The drawing under review shows one solid part. Ordinate dimensions are in mm from its lowest x, y, z. A direction names the side the tool comes from. Coordinates: 2 decimals unless noted, no trailing zeros. Write each loop counter-clockwise with the first axis right and the second up, starting at its lowest first coordinate (ties: lowest second). Pieces come first, ordered by that corner, then holes. Notation, with made-up numbers: M -1.5,-26.5 L 21.5,-26.5 A21 cw 21.5,-12.5 Z; hole C 10.5,19 d9. An arc over 180 degrees is marked long. Write each question's results on one line, items separated by ' | '. Start each with the question number.
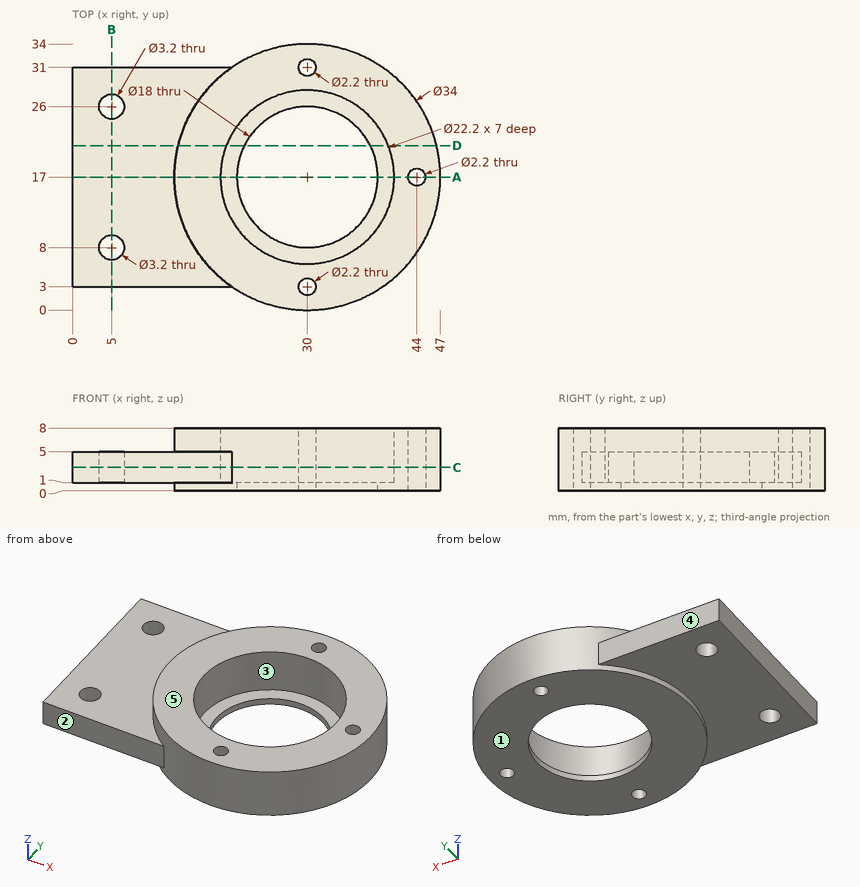
Item 1: For the marked faces 4 and 5, list the 3-axis set-ups (+Z, -Z, +X, -X, +Y, -Y) from which the entire face can be reached by the end or side of a thin tool; tool diameter is ignored.
Item 2: We need section A-A on y = 17. State the section outline as (x, z) points, then the cut area to 3 significant figures.
Item 3: We need section D-D on y = 21. State the section outline as (x, z) points.
Item 4: Draft analysis for pull direction Y (two halves, no side actions). For the marked faces 1, 2 and 3, state which applies: released by +Y, released by -Y, zero draft, split by the parting line, or undercut.
Item 5: Insertion check: pin 1 Ø1.5 at (y, z) = (20.5, 3.5) entering from +X; pin 2 Ø11 at (x, y) = (25.5, 14) entering from +Z; pin 3 Ø3 at (x, z) = (10, 3) entering from +Y. Each pin has a flat end and moves straight along its axis. Give the tip position at first contact, or say it passes through.
Item 6: Wall thickness on L1, parallel to Y at x = 30, z = 4; L2, parallel to Y at x = 5, z = 3.7; L3, parallel to Y at x = 30, z = 0.7: over which ranges is each line inside the solid? List them lowest first.
Item 7: We need section B-B on x = 5. State the section outline as (y, z) points.
Item 8: We need section C-C on z = 3. State the section outline as (x, y) points, then the cut area to 3 significant figures.
Answer:
1) face 4: +Z, -Z, -X, +Y | face 5: +Z, +X, -X, +Y, -Y
2) outline: M 0,1 L 13,1 L 13,0 L 21,0 L 21,1 L 18.9,1 L 18.9,8 L 13,8 L 13,5 L 0,5 Z; M 39,0 L 42.9,0 L 42.9,8 L 41.1,8 L 41.1,1 L 39,1 Z; M 45.1,0 L 47,0 L 47,8 L 45.1,8 Z | area: 133 mm^2
3) outline: M 0,1 L 13.48,1 L 13.48,0 L 21.94,0 L 21.94,1 L 19.65,1 L 19.65,8 L 13.48,8 L 13.48,5 L 0,5 Z; M 38.06,0 L 46.52,0 L 46.52,8 L 40.35,8 L 40.35,1 L 38.06,1 Z
4) face 1: zero draft | face 2: released by -Y | face 3: undercut
5) pin 1: stops at x = 46.78 | pin 2: stops at z = 1 | pin 3: stops at y = 31
6) L1: y = 0 to 1.9, 4.1 to 5.9, 28.1 to 29.9, 32.1 to 34 | L2: y = 3 to 6.4, 9.6 to 24.4, 27.6 to 31 | L3: y = 0 to 1.9, 4.1 to 8, 26 to 29.9, 32.1 to 34
7) outline: M 3,1 L 6.4,1 L 6.4,5 L 3,5 Z; M 9.6,1 L 24.4,1 L 24.4,5 L 9.6,5 Z; M 27.6,1 L 31,1 L 31,5 L 27.6,5 Z
8) outline: M 0,3 L 20.36,3 A17 ccw long 20.36,31 L 0,31 Z; hole C 5,8 d3.2; hole C 5,26 d3.2; hole C 30,17 d22.2; hole C 30,3 d2.2; hole C 30,31 d2.2; hole C 44,17 d2.2 | area: 919 mm^2
